Part model, mm, in its own coordinate system. Face numbers are marked on the shaded views. A direction names the side the tool comes from. Give positions to 0.01 mm unless a question says otherwise; leave off trailing zeros. Order: outer loops, then holes, each group sorted by start corner. A loop starts at its lowest first (then second) coordinate and runs counter-clockwise, first axis right, second up. Notation, with made-up numbers: M -31.75,6 L 17.25,6 A22 cw 17.25,17 Z; hole C -38.75,-21 d6. An arc over 180 degrees is marked long. Write each question's results on one line, items separated by ' | '. Start each with the question number.
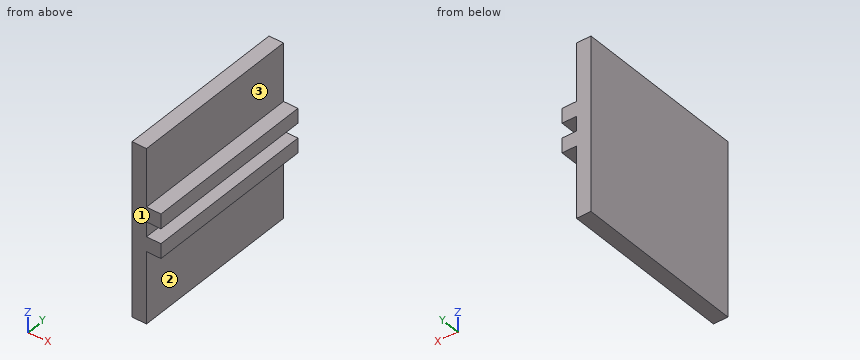
from build123d import *

# Parameters (mm, degrees)
F0_W     = 300
F0_H     = 300
F1_DEPTH = 25
F2_W     = 300
F2_H     = 25.4
F3_DEPTH = 25


with BuildPart() as f1:
    # F0 (on Right) → F1 (new body)
    with BuildSketch(Plane.YZ):
        Rectangle(F0_W, F0_H)
    extrude(amount=F1_DEPTH)

    # F2 (on face) → F3 (join)
    with BuildSketch(Plane.YZ.offset(25)):
        with Locations((0, -13.5)):
            Rectangle(F2_W, F2_H)
        with Locations((0, 37.3)):
            Rectangle(F2_W, F2_H)
    extrude(amount=F3_DEPTH)


solid = f1.part
(1) Saw through at A-A on x = 45.5. Give the cut face in (y, z), plus the area to 3 significant figures.
(2) Saw through at B-B on y = 31. Give the cut face in (x, z).
(3) Tool access for the marked faces 1, 2 and 3: list every direction of +Z, -Z, +X, -X, +Y, -Y with a clear straight run to the whole face (end or side of a thin tool).
(4) Drop flat-ended pins along their axis: P1, Ø1.5, axis at x = 32, y = -84.5, coming from the +Z side; P2, Ø7.5, axis at x = 38.5, y = -30, coming from the -Z side; P3, Ø10, axis at y = 118.5, z = -102.5, coming from the +X side. Give the stop position or say it passes through.
(5) Probe L1, parallel to Z at x = 27.5, y = 45.5; L2, parallel to X at y = 21, z = -78. List the from-to ranges inside material, lowest first.
(6) Saw through at C-C on z = -31. Give the cut face in (x, y).
Taken from the geometry:
1) outline: M -150,-26.2 L 150,-26.2 L 150,-0.8 L -150,-0.8 Z; M -150,24.6 L 150,24.6 L 150,50 L -150,50 Z | area: 15,200 mm²
2) outline: M 0,-150 L 25,-150 L 25,-26.2 L 50,-26.2 L 50,-0.8 L 25,-0.8 L 25,24.6 L 50,24.6 L 50,50 L 25,50 L 25,150 L 0,150 Z
3) face 1: +Z, -Z, +X, -X, -Y | face 2: -Z, +X, +Y, -Y | face 3: +Z, +X, +Y, -Y
4) P1: stops at z = 50 | P2: stops at z = -26.2 | P3: stops at x = 25
5) L1: z = -26.2 to -0.8, 24.6 to 50 | L2: x = 0 to 25
6) outline: M 0,-150 L 25,-150 L 25,150 L 0,150 Z
